Can you work these out from the model? Positions are in its coordinate system, mm. A direction names the side the tool comes from. Give positions to 0.01 mm unless a question says otherwise; leave off trailing zeros. Order: outer loops, then holes, each group sorted by start corner. A loop starts at its lowest first (then second) coordinate and runs counter-clockwise, first axis right, second up. Notation, with made-up numbers: (19.25, 0) -> (66.25, 0) arc R19 cw to (66.25, 33) -> close; hole circle Ø6 at (-16, 25). An arc over 180 degrees is marked (long way). Answer as a JSON object with one key per item and string values.
```python
from build123d import *

# Parameters (mm, degrees)
SKETCH2_R           = 2.5
BOSS_EXTRUDE1_DEPTH = 10
SKETCH9_W           = 10
SKETCH9_H           = 10
CUT_EXTRUDE1_DEPTH  = 4
SKETCH11_W          = 105
SKETCH11_H          = 93
CUT_EXTRUDE2_DEPTH  = 7
SKETCH12_W          = 5
SKETCH12_H          = 2
BOSS_EXTRUDE2_DEPTH = 2
SKETCH13_W          = 5
SKETCH13_H          = 5
BOSS_EXTRUDE3_DEPTH = 2


with BuildPart() as part:
    # Sketch2 → Boss-Extrude1 (new body)
    with BuildSketch(Plane(origin=(0, 0, 0), x_dir=(1, 0, 0), z_dir=(0, 1, 0))):
        Polygon((-59, 70), (-59, 49), (-80, 49), (-80, -49), (-59, -49), (-59, -70), (59, -70), (59, -49), (80, -49), (80, 49), (59, 49), (59, 70), align=None)
        with Locations(Location((0, 59.819243353, 0), (0, 0, 270))):
            Circle(SKETCH2_R, mode=Mode.SUBTRACT)
        with Locations(Location((0, -59.819243353, 0), (0, 0, 90))):
            Circle(SKETCH2_R, mode=Mode.SUBTRACT)
        with Locations(Location((-70, 0, 0), (0, 0, 270))):
            Circle(SKETCH2_R, mode=Mode.SUBTRACT)
        with Locations(Location((70, 0, 0), (0, 0, 90))):
            Circle(SKETCH2_R, mode=Mode.SUBTRACT)
    extrude(amount=BOSS_EXTRUDE1_DEPTH)

    # Sketch9 → Cut-Extrude1 (cut)
    with BuildSketch(Plane(origin=(0, 10, 0), x_dir=(1, 0, 0), z_dir=(0, 1, 0))):
        with Locations((0, 59.819243353)):
            Rectangle(SKETCH9_W, SKETCH9_H)
        with Locations((-70, 0)):
            Rectangle(SKETCH9_W, SKETCH9_H)
        with Locations((70, 0)):
            Rectangle(SKETCH9_W, SKETCH9_H)
        with Locations((0, -59.819243353)):
            Rectangle(SKETCH9_W, SKETCH9_H)
    extrude(amount=-CUT_EXTRUDE1_DEPTH, mode=Mode.SUBTRACT)

    # Sketch11 → Cut-Extrude2 (cut)
    with BuildSketch(Plane(origin=(0, 10, 0), x_dir=(1, 0, 0), z_dir=(0, 1, 0))):
        Rectangle(SKETCH11_W, SKETCH11_H)
    extrude(amount=-CUT_EXTRUDE2_DEPTH, mode=Mode.SUBTRACT)

    # Sketch12 → Boss-Extrude2 (add)
    with BuildSketch(Plane(origin=(0, 10, 0), x_dir=(1, 0, 0), z_dir=(0, 1, 0))):
        with Locations((-55, -44)):
            Rectangle(SKETCH12_W, SKETCH12_H)
        with Locations((55, -44)):
            Rectangle(SKETCH12_W, SKETCH12_H)
    extrude(amount=BOSS_EXTRUDE2_DEPTH)

    # Sketch13 → Boss-Extrude3 (add)
    with BuildSketch(Plane(origin=(0, 12, 0), x_dir=(1, 0, 0), z_dir=(0, 1, 0))):
        with Locations((-55, -44)):
            Rectangle(SKETCH13_W, SKETCH13_H)
        with Locations((55, -44)):
            Rectangle(SKETCH13_W, SKETCH13_H)
    extrude(amount=BOSS_EXTRUDE3_DEPTH)


solid = part.part
```
1. Will these pins go through, and if not, where does the flat tip stop? pin 1 Ø1.6 at (x, y) = (54, 13.5) entering from -Z; pin 2 Ø3 at (y, z) = (3.5, -64) entering from +X; pin 3 Ø3 at (x, z) = (0, -62) entering from +Y.
Worked answers:
{"pin 1": "z = 41.5", "pin 2": "x = 59", "pin 3": "y = 6"}
2. For faces 1 (the face through (59, 5, -59)), 2 (the face through (65, 8, 0)), 3 (the face through (-57.5, 12, 44)), 4 (the face through (-59, 5, -60)), which set-ups out of +Z, -Z, +X, -X, +Y, -Y let a thin tool reach every point of the face, with its end or its side?
Worked answers:
{"face 1": "-Z, +X, +Y, -Y", "face 2": "+Y", "face 3": "+Z, -Z, -X, +Y", "face 4": "-Z, -X, +Y, -Y"}
3. If we mould it in two halves opening along Z, with no side actions, what happens to faces 5 (the face through (75, 8, 0)), 6 (the face through (-70, 5, 49)), 7 (the face through (-59, 5, 59))? For each: +Z half, -Z half, draft (parallel to the pull), parting line (faces both ways), or undercut.
Worked answers:
{"face 5": "undercut", "face 6": "+Z half", "face 7": "draft"}
4. If we section it at B-B on z = 0: Please give me the cut outline in (x, y).
Worked answers:
{"outline": "(-80, 0) -> (-72.5, 0) -> (-72.5, 6) -> (-75, 6) -> (-75, 10) -> (-80, 10) -> close; (-67.5, 0) -> (67.5, 0) -> (67.5, 6) -> (65, 6) -> (65, 10) -> (52.5, 10) -> (52.5, 3) -> (-52.5, 3) -> (-52.5, 10) -> (-65, 10) -> (-65, 6) -> (-67.5, 6) -> close; (72.5, 0) -> (80, 0) -> (80, 10) -> (75, 10) -> (75, 6) -> (72.5, 6) -> close"}
5. If we section it at C-C on x = 0: Please give me the cut outline in (y, z).
Worked answers:
{"outline": "(0, -70) -> (10, -70) -> (10, -64.82) -> (6, -64.82) -> (6, -62.32) -> (0, -62.32) -> close; (0, -57.32) -> (6, -57.32) -> (6, -54.82) -> (10, -54.82) -> (10, -46.5) -> (3, -46.5) -> (3, 46.5) -> (10, 46.5) -> (10, 54.82) -> (6, 54.82) -> (6, 57.32) -> (0, 57.32) -> close; (0, 62.32) -> (6, 62.32) -> (6, 64.82) -> (10, 64.82) -> (10, 70) -> (0, 70) -> close"}
6. If we section it at D-D on x = 35.5: Please give me the cut outline in (y, z).
Worked answers:
{"outline": "(0, -70) -> (10, -70) -> (10, -46.5) -> (3, -46.5) -> (3, 46.5) -> (10, 46.5) -> (10, 70) -> (0, 70) -> close"}
7. Please list where these lines run through material, in increasing order: L1, parallel to X at y = 1.85, z = 0; L2, parallel to Z at x = 37.5, y = 6.25; L3, parallel to Z at x = 70, y = 1.45.
Worked answers:
{"L1": "-80 to -72.5, -67.5 to 67.5, 72.5 to 80", "L2": "-70 to -46.5, 46.5 to 70", "L3": "-49 to -2.5, 2.5 to 49"}
8. If we section it at A-A on x = 70: Please give me the cut outline in (y, z).
Worked answers:
{"outline": "(0, -49) -> (10, -49) -> (10, -5) -> (6, -5) -> (6, -2.5) -> (0, -2.5) -> close; (0, 2.5) -> (6, 2.5) -> (6, 5) -> (10, 5) -> (10, 49) -> (0, 49) -> close"}
